Here's how the part is built. I have some questions about the finished solid (model axes, mm). A direction names the side the tool comes from. Coordinates: 2 decimals unless noted, no trailing zeros. Write each loop counter-clockwise with the first axis right and the second up, starting at its lowest first coordinate (ties: lowest second). Pieces come first, ordered by that corner, then holes.
Item 1: Please list where these lines run through material, in increasing order: line 1 (Y direction, x = 2, z = -25.5); line 2 (X direction, y = -2.25, z = -23); line 3 (Z direction, x = -25.5, y = -7.5).
Item 2: I want a section at C-C (z = 0). Please give me the cut outline in (x, y) (3 decimals).
Item 3: I want a section at B-B (y = -9). Please give me the cut outline in (x, z).
Item 4: For faces 4 (the face through (20, -19.05, -26)), 5 (the face through (-23.493, -9.392, -23.088)), which set-ups out of +Z, -Z, +X, -X, +Y, -Y let a thin tool reach every point of the face, with its end or its side?
Item 5: If we mould it in two halves opening along X, with no side actions, what happens to faces 1 (the face through (11, -19.05, 31)), 2 (the face through (17.6, -9.4, -28.8)), 3 (the face through (-42.773, 0.196, -9.498))? For each: pulls with the +X half, pulls with the -X half, needs draft (parallel to the pull), parting line crosses it, or undercut.
Item 6: I'm going to push flat-ended pins straight in: P1, Ø6, axis at x = -27, y = -12, coming from the -Z side; P2, Ø6, axis at x = -22.5, z = -6, coming from the -Y side; P3, Ø10, axis at y = -9.5, z = 32.5, coming from the -X side. Where does each tip first touch, or does it pass through?
Item 7: I want a section at A-A (x = 20.32). Please give me the cut outline in (y, z), and give its area (3 significant figures).
Item 8: I want a section at D-D (x = -27). Please give me the cut outline in (y, z).
from build123d import *

# Parameters (mm, degrees)
SKETCH1_R           = 43.815
BOSS_EXTRUDE1_DEPTH = 0.396875
SKETCH2_R           = 3.96875
BOSS_EXTRUDE2_DEPTH = 19.05


with BuildPart() as part:
    # Sketch1 → Boss-Extrude1 (new body)
    with BuildSketch(Plane(origin=(0, 0, 0), x_dir=(1, 0, 0), z_dir=(0, 1, 0))):
        with Locations(Location((0, 0, 0), (0, 0, 270))):
            Circle(SKETCH1_R)
    extrude(amount=BOSS_EXTRUDE1_DEPTH)

    # Sketch2 → Boss-Extrude2 (add)
    with BuildSketch(Plane.XZ):
        with Locations(Location((20.32, -25.908, 0), (0, 0, 90))):
            Circle(SKETCH2_R)
        with Locations(Location((-25.908, -19.939, 0), (0, 0, 90))):
            Circle(SKETCH2_R)
        with Locations(Location((10.668, 30.861, 0), (0, 0, 90))):
            Circle(SKETCH2_R)
    extrude(amount=BOSS_EXTRUDE2_DEPTH)


solid = part.part
Answer:
1. line 1: y = 0 to 0.4
1. line 2: x = -28.43 to -23.38, 17.62 to 23.02
1. line 3: z = -23.89 to -15.99
2. outline: (-43.815, 0) - (43.815, 0) - (43.815, 0.397) - (-43.815, 0.397) - close
3. outline: circle Ø7.94 at (-25.91, -19.94); circle Ø7.94 at (10.67, 30.86); circle Ø7.94 at (20.32, -25.91)
4. face 4: +Z, -Z, +X, -X, -Y
4. face 5: -Y
5. face 1: needs draft
5. face 2: undercut
5. face 3: parting line crosses it
6. P1: stops at z = -23.91
6. P2: stops at y = 0
6. P3: stops at x = 6.7
7. outline: (-19.05, -29.88) - (0, -29.88) - (0, -38.82) - (0.4, -38.82) - (0.4, 38.82) - (0, 38.82) - (0, -21.94) - (-19.05, -21.94) - close
7. area: 182 mm2
8. outline: (-19.05, -23.75) - (0, -23.75) - (0, -34.51) - (0.4, -34.51) - (0.4, 34.51) - (0, 34.51) - (0, -16.12) - (-19.05, -16.12) - close
